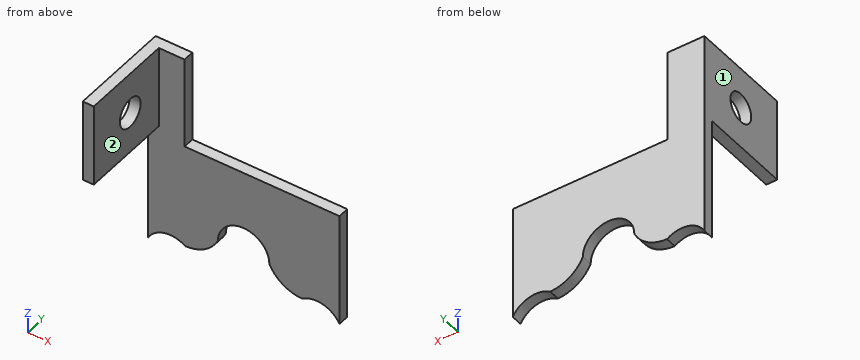
from build123d import *

# Parameters (mm, degrees)
BOSS_EXTRUDE1_DEPTH = 3
SKETCH3_W           = 10
SKETCH3_H           = 3
BOSS_EXTRUDE2_DEPTH = 25
SKETCH4_W           = 3
SKETCH4_H           = 22.5
BOSS_EXTRUDE3_DEPTH = 25
SKETCH5_R           = 4
CUT_EXTRUDE1_DEPTH  = 3


with BuildPart() as part:
    # Sketch2 → Boss-Extrude1 (new body)
    with BuildSketch(Plane(origin=(0, 0, 0), x_dir=(1, 0, 0), z_dir=(0, 1, 0))):
        with BuildLine():
            Line((26.055569119, 8.188046441), (26.055569119, -22.834953559))
            Line((26.055569119, -22.834953559), (-26.055569119, -22.834953559))
            Line((-26.055569119, -22.834953559), (-26.055569119, 8.188046441))
            ThreePointArc((-26.055569119, 8.188046441), (-21.514872246, 4.669726518), (-15.870079226, 5.73406431))
            ThreePointArc((-15.870079226, 5.73406431), (-10.616247764, 4.133629141), (-7, 0))
            ThreePointArc((-7, 0), (0, -7), (7, 0))
            ThreePointArc((7, 0), (10.616247764, 4.133629141), (15.870079226, 5.73406431))
            ThreePointArc((15.870079226, 5.73406431), (21.514872246, 4.669726518), (26.055569119, 8.188046441))
        make_face()
    extrude(amount=BOSS_EXTRUDE1_DEPTH)

    # Sketch3 → Boss-Extrude2 (add)
    with BuildSketch(Plane.XY.offset(22.834953559)):
        with Locations((-21.055569119, 1.5)):
            Rectangle(SKETCH3_W, SKETCH3_H)
    extrude(amount=BOSS_EXTRUDE2_DEPTH)

    # Sketch4 → Boss-Extrude3 (add)
    with BuildSketch(Plane.XZ):
        with Locations((-24.555569119, 36.584953559)):
            Rectangle(SKETCH4_W, SKETCH4_H)
    extrude(amount=BOSS_EXTRUDE3_DEPTH)

    # Sketch5 → Cut-Extrude1 (cut)
    with BuildSketch(Plane.ZY.offset(26.055569119)):
        with Locations((36.584953559, -11)):
            Circle(SKETCH5_R)
    extrude(amount=-CUT_EXTRUDE1_DEPTH, mode=Mode.SUBTRACT)


solid = part.part
Read the model definition and answer for the solid it produces. Units are mm, in the model's axes. Face numbers are marked on the shaded views. A direction names the side the tool comes from. Round coordinates to 2 decimals unless told otherwise and drop trailing zeros. Order: outer loops, then holes, each group sorted by start corner. A loop starts at its lowest first (then second) coordinate and runs counter-clockwise, first axis right, second up.
1) The part is cut by section C-C on x = 0. Write down the section's boundary in (y, z).
2) Straight lines are drawn through the part: L1, parallel to Y at x = 12, z = 11; L2, parallel to X at y = -1, z = 27.5. For each, find the intervals that lie inside material, in ascending order.
3) The part is cut by section B-B on z = -2.5. Write down the section's boundary in (x, y), plus the area to 3 significant figures.
4) The part is cut by section A-A on y = -12.25. Write down the section's boundary in (x, z).
5) Flat-ended cylindrical pins translate along their axes: pin 1 (0.9 mm diameter, centred on x = 8, y = 1, fed in from +Z); pin 2 (3.5 mm diameter, centred on y = 1.5, z = 35.5, fed in from +X); pin 3 (3 mm diameter, centred on x = -11.5, z = 26, fed in from +Y); pin 4 (11 mm diameter, centred on y = -17, z = 40, fed in from +X). Find the tip coordinate at first contact, or state that the pin passes through.
6) The part is cut by section D-D on z = 38. Write down the section's boundary in (x, y), plus the area to 3 significant figures.
7) For the marked faces 1 and 2, determine the directions among +Z, -Z, +X, -X, +Y, -Y from which every point of the face is accessible in a straight line to the end or side of a thin tool.
Resolved:
1. outline: (0, 7) - (3, 7) - (3, 22.83) - (0, 22.83) - close
2. L1: y = 0 to 3
2. L2: x = -26.06 to -23.06
3. outline: (-26.06, 0) - (-8.68, 0) - (-8.68, 3) - (-26.06, 3) - close; (8.68, 0) - (26.06, 0) - (26.06, 3) - (8.68, 3) - close
3. area: 104 mm2
4. outline: (-26.06, 25.33) - (-23.06, 25.33) - (-23.06, 32.79) - (-26.06, 32.79) - close; (-26.06, 40.38) - (-23.06, 40.38) - (-23.06, 47.83) - (-26.06, 47.83) - close
5. pin 1: stops at z = 22.83
5. pin 2: stops at x = -16.06
5. pin 3: passes through
5. pin 4: stops at x = -23.06
6. outline: (-26.06, -25) - (-23.06, -25) - (-23.06, -14.74) - (-26.06, -14.74) - close; (-26.06, -7.26) - (-23.06, -7.26) - (-23.06, 0) - (-16.06, 0) - (-16.06, 3) - (-26.06, 3) - close
6. area: 82.6 mm2
7. face 1: +Z, -Z, -X, +Y, -Y
7. face 2: +Z, -Z, +X, -Y
